For this review, use the dimensioned drawing (mm, ordinates from the lowest corner) and the shaded views. Coordinates: 2 decimals unless noted, no trailing zeros. Order: outer loops, then holes, each group sorted by start corner. A loop starts at its lowest first (then second) coordinate and runs counter-clockwise, first axis right, second up. Notation, with made-up numbers: (65, 67.5) -> (109, 67.5) arc R12 cw to (109, 79.5) -> close; hole circle Ø3 at (-17.75, -21). An arc over 180 degrees is marked (long way). Return JSON: item names as keys, results as strings. Group by question number.
Item 1: Take a section at B-B (y = 305.5). Write out the cut boundary in (x, z).
Item 2: For line 1 along X through (y, z) = (279.5, 5.75); line 2 along Y through (x, z) = (733.5, 14); line 3 along X through (y, z) = (323, 14), list the stretches that pass through material, from the lowest coordinate up.
Item 3: Insertion check: pin 1 (6.5 mm diameter, centred on y = 391, z = 6, fed in from +X); pin 2 (1.5 mm diameter, centred on x = 664, z = 4, fed in from +Y); pin 3 (2 mm diameter, centred on x = 798.5, z = 16.5, fed in from -Y). Each pin has a flat end and moves straight along its axis. Give the tip position at first contact, or say it passes through.
Item 4: Take a section at A-A (z = 15.75). Write out the cut boundary in (x, y), then the cut area to 3 significant figures.
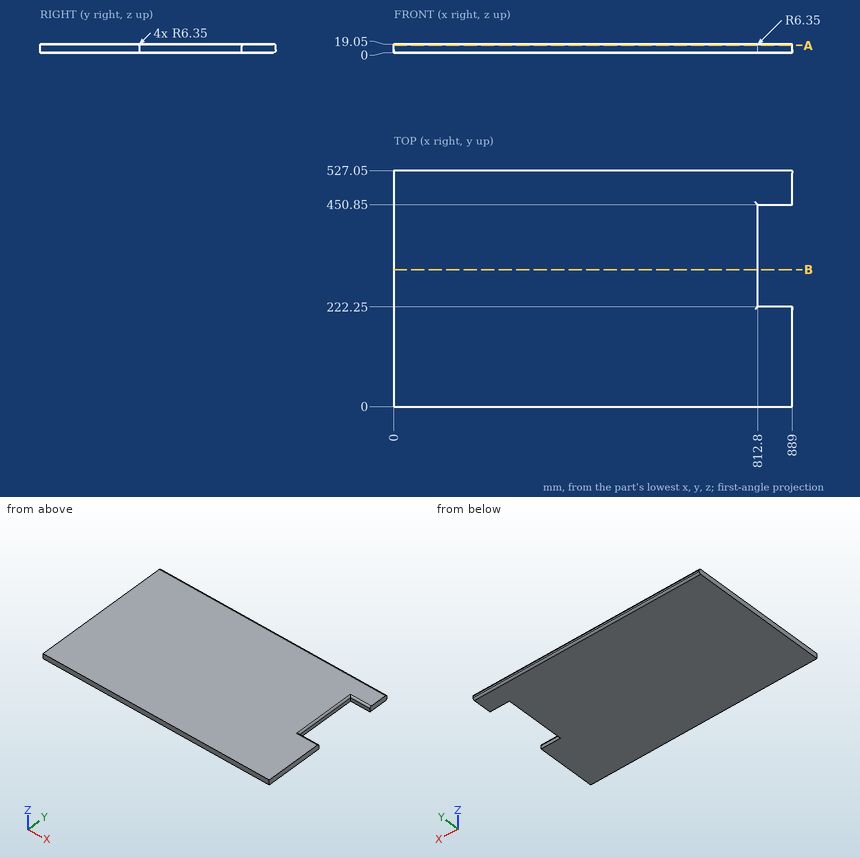
Findings below:
{
 "1": {"outline": "(0, 0) -> (812.8, 0) -> (812.8, 12.7) arc R6.35 ccw to (806.45, 19.05) -> (0, 19.05) -> close"},
 "2": {"line 1": "x = 0 to 812.8", "line 2": "y = 0 to 526.92", "line 3": "x = 0 to 812.67"},
 "3": {"pin 1": "stops at x = 812.8", "pin 2": "stops at y = 526.85", "pin 3": "stops at y = 0"},
 "4": {"outline": "(0, 0) -> (889, 0) -> (889, 221.47) -> (812.02, 221.47) -> (812.02, 451.63) -> (889, 451.63) -> (889, 526.27) -> (0, 526.27) -> close", "area": "450,000 mm2"}
}
